Autodesk Inventor part; units mm, degrees
ref_plane "YZ Plane" through (0, 0, 0) normal (1, 0, 0) x (0, 1, 0)
ref_plane "XZ Plane" through (0, 0, 0) normal (0, 1, 0) x (-1, 0, 0)
ref_plane "XY Plane" through (0, 0, 0) normal (0, 0, 1) x (1, 0, 0)
sketch "Sketch2" plane through (0, 0, 0) normal (0, 1, 0) x (-1, 0, 0)
  circle A0 centre (0, 0) radius 8.9778 construction
  circle A1 centre (0, 0) radius 6.9178 construction
  arc A2 (0, -6.9178) -> (-1.5221, -8.3486) centre (0, -8.4428) ccw
  line L0 (0, 0) -> (0, -8.9778) construction
  line L1 (0, 0) -> (-2.3236, -8.6719) construction
  arc A3 (-2.0494, -8.7407) -> (-1.5221, -8.3486) centre (-1.9513, -8.3221) ccw
  arc A4 (-2.8562, -7.9912) -> (-3.4589, -5.991) centre (-4.2214, -7.3117) ccw
  arc A5 (-2.8562, -7.9912) -> (-2.5955, -8.5944) centre (-2.4712, -8.1828) ccw
  arc A6 (-2.5955, -8.5944) -> (-2.0494, -8.7407) centre (0, 0) ccw
  arc A7 (2.5955, -8.5944) -> (2.8562, -7.9912) centre (2.4712, -8.1828) ccw
  arc A8 (1.5221, -8.3486) -> (0, -6.9178) centre (0, -8.4428) ccw
  arc A9 (1.5221, -8.3486) -> (2.0494, -8.7407) centre (1.9513, -8.3221) ccw
  arc A10 (2.0494, -8.7407) -> (2.5955, -8.5944) centre (0, 0) ccw
  arc A11 (3.4589, -5.991) -> (2.8562, -7.9912) centre (4.2214, -7.3117) ccw
  arc A12 (6.545, -6.1452) -> (6.4691, -5.4925) centre (6.2315, -5.8509) ccw
  arc A13 (5.4925, -6.4691) -> (3.4589, -5.991) centre (4.2214, -7.3117) ccw
  arc A14 (5.4925, -6.4691) -> (6.1452, -6.545) centre (5.8509, -6.2315) ccw
  arc A15 (6.1452, -6.545) -> (6.545, -6.1452) centre (0, 0) ccw
  arc A16 (5.991, -3.4589) -> (6.4691, -5.4925) centre (7.3117, -4.2214) ccw
  arc A17 (8.7407, -2.0494) -> (8.3486, -1.5221) centre (8.3221, -1.9513) ccw
  arc A18 (7.9912, -2.8562) -> (5.991, -3.4589) centre (7.3117, -4.2214) ccw
  arc A19 (7.9912, -2.8562) -> (8.5944, -2.5955) centre (8.1828, -2.4712) ccw
  arc A20 (8.5944, -2.5955) -> (8.7407, -2.0494) centre (0, 0) ccw
  arc A21 (6.9178, 0) -> (8.3486, -1.5221) centre (8.4428, 0) ccw
  arc A22 (8.5944, 2.5955) -> (7.9912, 2.8562) centre (8.1828, 2.4712) ccw
  arc A23 (8.3486, 1.5221) -> (6.9178, 0) centre (8.4428, 0) ccw
  arc A24 (8.3486, 1.5221) -> (8.7407, 2.0494) centre (8.3221, 1.9513) ccw
  arc A25 (8.7407, 2.0494) -> (8.5944, 2.5955) centre (0, 0) ccw
  arc A26 (5.991, 3.4589) -> (7.9912, 2.8562) centre (7.3117, 4.2214) ccw
  arc A27 (6.1452, 6.545) -> (5.4925, 6.4691) centre (5.8509, 6.2315) ccw
  arc A28 (6.4691, 5.4925) -> (5.991, 3.4589) centre (7.3117, 4.2214) ccw
  arc A29 (6.4691, 5.4925) -> (6.545, 6.1452) centre (6.2315, 5.8509) ccw
  arc A30 (6.545, 6.1452) -> (6.1452, 6.545) centre (0, 0) ccw
  arc A31 (3.4589, 5.991) -> (5.4925, 6.4691) centre (4.2214, 7.3117) ccw
  arc A32 (2.0494, 8.7407) -> (1.5221, 8.3486) centre (1.9513, 8.3221) ccw
  arc A33 (2.8562, 7.9912) -> (3.4589, 5.991) centre (4.2214, 7.3117) ccw
  arc A34 (2.8562, 7.9912) -> (2.5955, 8.5944) centre (2.4712, 8.1828) ccw
  arc A35 (2.5955, 8.5944) -> (2.0494, 8.7407) centre (0, 0) ccw
  arc A36 (0, 6.9178) -> (1.5221, 8.3486) centre (0, 8.4428) ccw
  arc A37 (-2.5955, 8.5944) -> (-2.8562, 7.9912) centre (-2.4712, 8.1828) ccw
  arc A38 (-1.5221, 8.3486) -> (0, 6.9178) centre (0, 8.4428) ccw
  arc A39 (-1.5221, 8.3486) -> (-2.0494, 8.7407) centre (-1.9513, 8.3221) ccw
  arc A40 (-2.0494, 8.7407) -> (-2.5955, 8.5944) centre (0, 0) ccw
  arc A41 (-3.4589, 5.991) -> (-2.8562, 7.9912) centre (-4.2214, 7.3117) ccw
  arc A42 (-6.545, 6.1452) -> (-6.4691, 5.4925) centre (-6.2315, 5.8509) ccw
  arc A43 (-5.4925, 6.4691) -> (-3.4589, 5.991) centre (-4.2214, 7.3117) ccw
  arc A44 (-5.4925, 6.4691) -> (-6.1452, 6.545) centre (-5.8509, 6.2315) ccw
  arc A45 (-6.1452, 6.545) -> (-6.545, 6.1452) centre (0, 0) ccw
  arc A46 (-5.991, 3.4589) -> (-6.4691, 5.4925) centre (-7.3117, 4.2214) ccw
  arc A47 (-8.7407, 2.0494) -> (-8.3486, 1.5221) centre (-8.3221, 1.9513) ccw
  arc A48 (-7.9912, 2.8562) -> (-5.991, 3.4589) centre (-7.3117, 4.2214) ccw
  arc A49 (-7.9912, 2.8562) -> (-8.5944, 2.5955) centre (-8.1828, 2.4712) ccw
  arc A50 (-8.5944, 2.5955) -> (-8.7407, 2.0494) centre (0, 0) ccw
  arc A51 (-6.9178, 0) -> (-8.3486, 1.5221) centre (-8.4428, 0) ccw
  arc A52 (-8.5944, -2.5955) -> (-7.9912, -2.8562) centre (-8.1828, -2.4712) ccw
  arc A53 (-8.3486, -1.5221) -> (-6.9178, 0) centre (-8.4428, 0) ccw
  arc A54 (-8.3486, -1.5221) -> (-8.7407, -2.0494) centre (-8.3221, -1.9513) ccw
  arc A55 (-8.7407, -2.0494) -> (-8.5944, -2.5955) centre (0, 0) ccw
  arc A56 (-5.991, -3.4589) -> (-7.9912, -2.8562) centre (-7.3117, -4.2214) ccw
  arc A57 (-6.1452, -6.545) -> (-5.4925, -6.4691) centre (-5.8509, -6.2315) ccw
  arc A58 (-6.4691, -5.4925) -> (-5.991, -3.4589) centre (-7.3117, -4.2214) ccw
  arc A59 (-6.4691, -5.4925) -> (-6.545, -6.1452) centre (-6.2315, -5.8509) ccw
  arc A60 (-6.545, -6.1452) -> (-6.1452, -6.545) centre (0, 0) ccw
  arc A61 (-3.4589, -5.991) -> (-5.4925, -6.4691) centre (-4.2214, -7.3117) ccw
  point P0 (2.3236, -8.6719)
  point P1 (6.3483, -6.3483)
  point P2 (8.6719, -2.3236)
  point P3 (8.6719, 2.3236)
  point P4 (6.3483, 6.3483)
  point P5 (2.3236, 8.6719)
  point P6 (-2.3236, 8.6719)
  point P7 (-6.3483, 6.3483)
  point P8 (-8.6719, 2.3236)
  point P9 (3.4589, -5.991)
  point P10 (6.9178, 0)
  point P11 (5.991, 3.4589)
  point P12 (3.4589, 5.991)
  point P13 (0, 6.9178)
  point P14 (-5.991, 3.4589)
  point P15 (-3.1307, -4.309)
  point P16 (0, -6.9178)
  point P17 (-8.6719, -2.3236)
  point P18 (-6.3483, -6.3483)
  dimension "d1" = 13.8356
  dimension "d2" = 17.9556
  dimension "d3" = 15
  dimension "d4" = 3.05
  dimension "d5" = 0.86
  dimension "d8" = 360
extrude "Extrusion1" add sketch "Sketch2" along normal blind 9
properties part number "5mm_HTD_Pully"
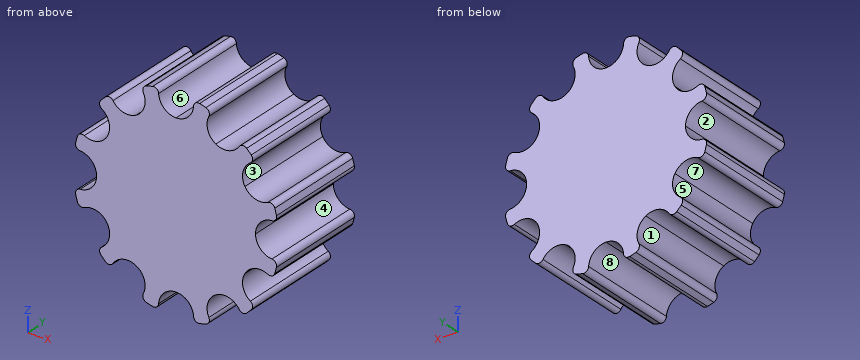
Verification items for the finished model (mm, model axes). Face numbers are marked on the shaded views. A direction names the side the tool comes from. Give positions to 0.01 mm unless a question says otherwise; leave off trailing zeros. Order: outer loops, then holes, each group sorted by start corner. A loop starts at its lowest first (then second) coordinate and runs counter-clockwise, first axis right, second up. Notation, with made-up numbers: (4.25, -5) - (18.25, -5) arc R34 cw to (18.25, 25) - close; hole circle Ø2 at (17.5, 67.5). An arc over 180 degrees is marked (long way). Answer as CSV lines item,"result". Start each with the question number.
Item 1: Section check A-A, the plane x = 4.25. Record the boundary of the cut face in (y, z).
Item 2: Material ranges on L1, parallel to Z at x = -6, y = 4.75; L2, parallel to Z at x = 4.25, y = 2, recorded low to high.
Item 3: Mould release check, pull along X, two halves, no side actions. Record for the marked faces 1, 2 and 3: released by +X, released by -X, zero draft, split by the parting line, or undercut.
Item 4: Access from +Z, -Z, +X, -X, +Y, -Y to the whole of each face (thin tool, end or side, straight path). Record for the marked faces 4, 5, 6, 7 and 8.
Item 5: Section check B-B, the plane z = -4.5. Record the boundary of the cut face in (x, y), plus the area to 3 significant figures.
Item 6: Gauge pin test, flat end, axial feed: pin 1 (1.5 mm diameter, centred on x = -7, y = 6.5, fed in from -Z) (3 decimals). Record the tip position at first contact, or that the pin passes through.
Filled in:
1,outline,"(0, -5.79) - (9, -5.79) - (9, 5.79) - (0, 5.79) - close"
2,L1,"-6.63 to -5, -3.44 to 3.44, 5 to 6.63"
2,L2,"-5.79 to 5.79"
3,face 1,"undercut"
3,face 2,"released by -X"
3,face 3,"released by +X"
4,face 4,"+X, +Y, -Y"
4,face 5,"-X, +Y, -Y"
4,face 6,"+Z, +Y, -Y"
4,face 7,"+Y, -Y"
4,face 8,"-Z, +Y, -Y"
5,outline,"(-5.81, 0) - (5.81, 0) - (5.81, 9) - (-5.81, 9) - close"
5,area,"105 mm^2"
6,pin 1,"z = -6.445"
